Design review of the part shown in the three views and the two pictorial views. Dimensions are in mm from the part's minimum x, y and z. A direction names the side the tool comes from. Coordinates: 2 decimals unless noted, no trailing zeros. Order: outer loops, then holes, each group sorted by start corner. A loop starts at its lowest first (then second) coordinate and runs counter-clockwise, first axis right, second up. Notation, with made-up numbers: (-29, 74.5) -> (-12, 74.5) arc R19 cw to (-12, 87.5) -> close; hole circle Ø7 at (-12.75, 78.25). An arc over 180 degrees is marked (long way). Answer as a JSON object with one key per item and string values. Group by question number.
1) Machinability: for the marked faces 1, 2 and 3, which of the approach directions +Z, -Z, +X, -X, +Y, -Y give a long, thin tool a straight path to every point of the face, cutting with its end or side? Answer none if there is none.
2) Add section B-B, the plane x = 17. Write out the cut boundary in (y, z).
3) Add section A-A, the plane y = 7.25. Write out the cut boundary in (x, z), then the cut area to 3 significant figures.
4) Wall thickness on L1, parallel to Z at x = 43, y = 3.2; L2, parallel to X at y = 21.75, z = 16.5; L3, parallel to Z at x = 15, y = 26.25: over which ranges is each line inside the solid? List them lowest first.
5) Add section C-C, the plane z = 59. Write out the cut boundary in (x, y), then the cut area to 3 significant figures.
6) For pin 1 (5 mm diameter, centred on x = 13, y = 19, fed in from -Z); pin 2 (4 mm diameter, centred on y = 23.5, z = 76, fed in from -X); pin 3 (10 mm diameter, centred on x = 7.5, y = 4.5, fed in from +Z), all flat-tipped, find the tip position at first contact; note any pin that passes through.
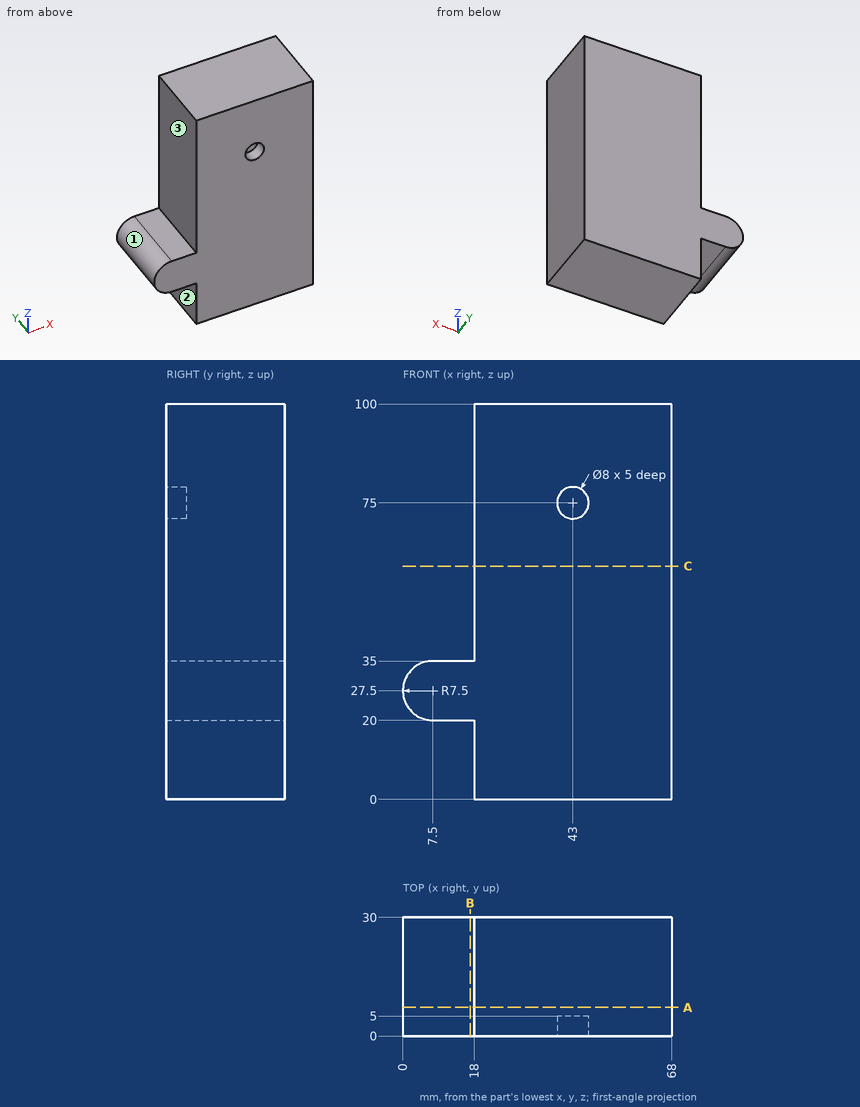
Output values:
{
 "1": {"face 1": "-X, +Y, -Y", "face 2": "-Z, -X, +Y, -Y", "face 3": "+Z, -X, +Y, -Y"},
 "2": {"outline": "(0, 20) -> (30, 20) -> (30, 35) -> (0, 35) -> close"},
 "3": {"outline": "(7.5, 20) -> (18, 20) -> (18, 0) -> (68, 0) -> (68, 100) -> (18, 100) -> (18, 35) -> (7.5, 35) arc R7.5 ccw to start", "area": "5,250 mm²"},
 "4": {"L1": "z = 0 to 71, 79 to 100", "L2": "x = 18 to 68", "L3": "z = 20 to 35"},
 "5": {"outline": "(18, 0) -> (68, 0) -> (68, 30) -> (18, 30) -> close", "area": "1,500 mm²"},
 "6": {"pin 1": "stops at z = 20", "pin 2": "stops at x = 18", "pin 3": "stops at z = 35"}
}
